Work out the finished part from the listing and answer in its coordinate system (mm). Face numbers are marked on the shaded views. Give positions to 0.01 mm unless a question says otherwise; leave off trailing zeros. Write each loop counter-clockwise with the first axis right and the second up, starting at its lowest first coordinate (ties: lowest second). Pieces come first, ordered by that corner, then holes. Notation, with made-up numbers: (-30, 75) -> (-21, 75) arc R14 ccw to (-21, 98) -> close; hole circle Ø7 at (-39, 29). An arc over 180 degrees is marked (long way). Use a Markdown table: item, result. Add a question column.
Q1. Consider line 1 (Y direction, x = 12, z = 7); line 2 (X direction, y = 1.55, z = -6.75); line 3 (Z direction, x = -8, y = 1.7). Determine where each line is inside the solid, lowest interval first.
Q2. Section C-C, the plane y = 0.4 is taken. Give the vertices of the cut face in (x, z).
Q3. Each of these flat-tipped pins is pushed along its axis until it touches: pin 1 Ø3 at (x, z) = (0, 9) entering from -Y; pin 2 Ø1 at (x, y) = (6, 0.5) entering from +Z; pin 3 Ø1 at (y, z) = (0, 9.5) entering from +X; pin 4 Ø2 at (x, y) = (-9.5, 0.5) entering from +Z. Where does it stop, or does it pass through?
Q4. For a pull along X with two mould halves and no side action, classify the marked faces 1, 2 and 3 as pulls with the +X half, pulls with the -X half, needs draft (parallel to the pull), parting line crosses it, or undercut.
Q5. Section A-A, the plane x = 0 is taken. Give the vertices of the cut face in (y, z), plus the area to 3 significant figures.
Q6. Section B-B, the plane z = 0 is taken. Give the vertices of the cut face in (x, y).
from build123d import *

# Parameters (mm, degrees)
SKETCH003_R        = 1.5
SKETCH_R           = 15
PAD_DEPTH          = 2.5
SKETCH005_R        = 2
POCKET001_DEPTH    = 90.441037
POLARPATTERN_COUNT = 5


with BuildPart() as body001:
    # AdditivePipe: sweep along a path in Sketch002
    with BuildLine(Plane.XZ) as additivepipe_path:
        CenterArc((0, 0), 9, 0, 360)
    # Sketch003 → AdditivePipe (sweep)
    with BuildSketch(Plane.XY):
        with Locations((-14, 0)):
            Circle(SKETCH003_R)
    sweep(path=additivepipe_path.line)


with BuildPart() as cut:
    # Sketch → Pad (new body, symmetric)
    with BuildSketch(Plane.XZ):
        Circle(SKETCH_R)
    extrude(amount=PAD_DEPTH, both=True)

    # Sketch005 → Pocket001 (cut, through all)
    with BuildSketch(Plane.XZ.offset(2.5)):
        with Locations((0, 9)):
            Circle(SKETCH005_R)
    pocket001 = extrude(amount=-POCKET001_DEPTH, mode=Mode.SUBTRACT)

    # PolarPattern: Pocket001 ×5 about axis
    polarpattern_axis = Axis((0, -2.5, 0), (0, -1, 0))
    for i in range(1, POLARPATTERN_COUNT):
        add(pocket001.rotate(polarpattern_axis, i * 360 / POLARPATTERN_COUNT), mode=Mode.SUBTRACT)

    # Cut: cut Body001
    add(body001.part, mode=Mode.SUBTRACT)


solid = cut.part
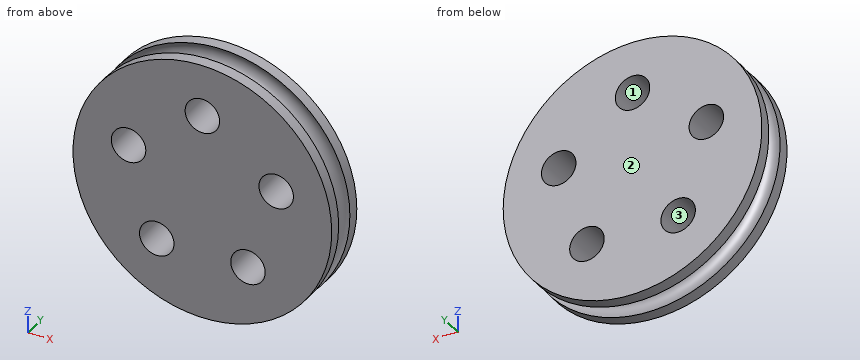
Result set:
| question | item | result |
|---|---|---|
| 1 | line 1 | y = -2.5 to -1.5, 1.5 to 2.5 |
| 1 | line 2 | x = -13.4 to -7.22, -3.36 to 3.36, 7.22 to 13.4 |
| 1 | line 3 | z = -12.69 to 0.86, 4.7 to 12.69 |
| 2 | outline | circle Ø25.11 at (0, 0); hole circle Ø4 at (-8.56, 2.78); hole circle Ø4 at (-5.29, -7.28); hole circle Ø4 at (0, 9); hole circle Ø4 at (5.29, -7.28); hole circle Ø4 at (8.56, 2.78) |
| 3 | pin 1 | passes through |
| 3 | pin 2 | stops at z = 11.46 |
| 3 | pin 3 | stops at x = 8.67 |
| 3 | pin 4 | stops at z = 12.21 |
| 4 | face 1 | undercut |
| 4 | face 2 | needs draft |
| 4 | face 3 | undercut |
| 5 | outline | (-2.5, -15) -> (-1.12, -15) arc R1.5 cw (long way) to (1.12, -15) -> (2.5, -15) -> (2.5, 7) -> (-2.5, 7) -> close; (-2.5, 11) -> (2.5, 11) -> (2.5, 15) -> (1.12, 15) arc R1.5 cw (long way) to (-1.12, 15) -> (-2.5, 15) -> close |
| 5 | area | 117 mm2 |
| 6 | outline | (-15, -2.5) -> (15, -2.5) -> (15, -1.12) arc R1.5 cw (long way) to (15, 1.12) -> (15, 2.5) -> (-15, 2.5) -> (-15, 1.12) arc R1.5 cw (long way) to (-15, -1.12) -> close |
